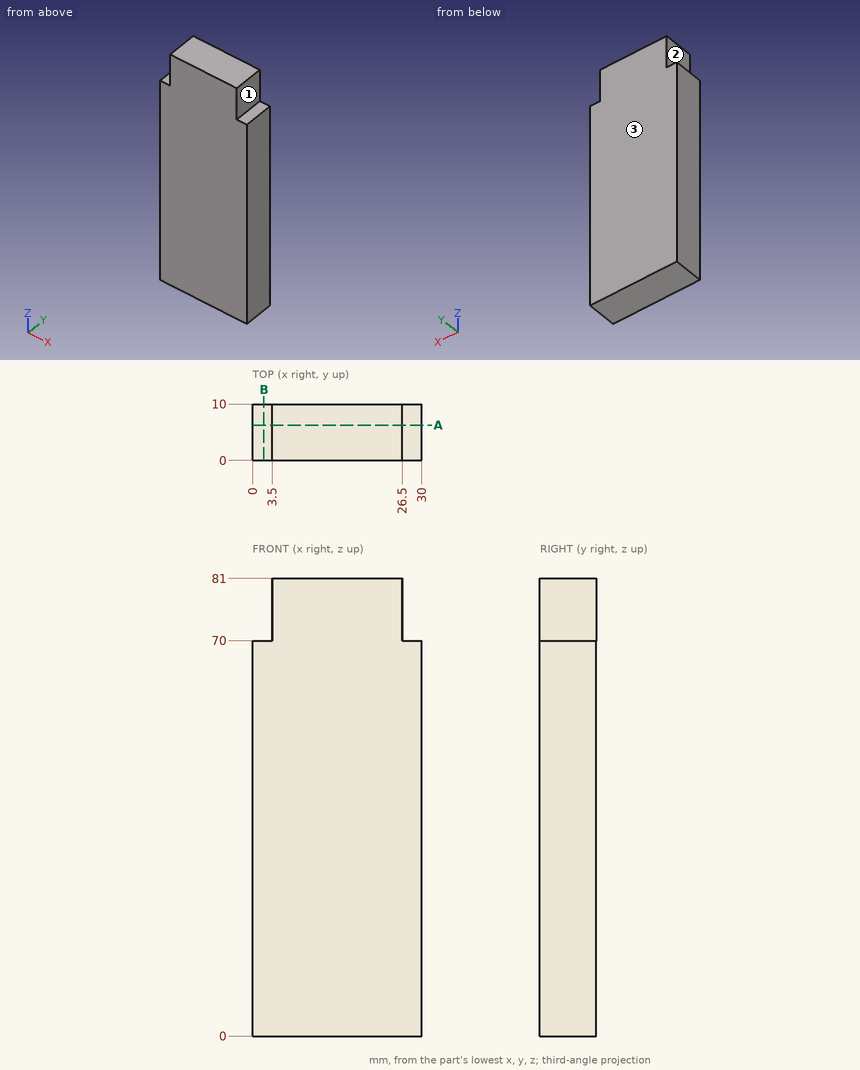
The figure shows three views and two pictorial views of one solid part (mm, origin at its lowest corner). Answer the questions. A direction names the side the tool comes from. Give positions to 0.01 mm unless a question says otherwise; leave off trailing zeros. Loops run counter-clockwise (first coordinate to the right, second up) from the corner with the lowest first, then second, coordinate; pieces in that order, holes last. Notation, with made-up numbers: (-26.5, 74.25) -> (22.5, 74.25) arc R29 ccw to (22.5, 102.25) -> close; hole circle Ø8 at (29.5, 17.5). An arc over 180 degrees is marked (long way). Put each result on its own line as item: value. Start each with the question number.
Item 1: Which of the six approach directions +Z, -Z, +X, -X, +Y, -Y give full straight-line access (tool end or side, diameter ignored) to the marked faces 1, 2 and 3?
Item 2: The part is cut by section A-A (y = 6.25). Give the vertices of the cut face in (x, z), then the cut area to 3 significant figures.
Item 3: Find the intervals of material crossed by L1, parallel to Z at x = 27.5, y = 8.5; L2, parallel to X at y = 3, z = 70.5, in increasing order. Write a range as [from, to].
Item 4: Each of these flat-tipped pins is pushed along its axis until it touches: P1, Ø4, axis at x = 29, y = 3, coming from the +Z side; P2, Ø5, axis at y = 2.5, z = 74, coming from the -X side. Where does it stop, or does it pass through?
Item 5: The part is cut by section B-B (x = 2). Give the vertices of the cut face in (y, z).
Answers below:
1. face 1: +Z, +X, +Y, -Y
1. face 2: +Z, -X, +Y, -Y
1. face 3: +Z, -Z, +X, -X, +Y
2. outline: (0, 0) -> (30, 0) -> (30, 70) -> (26.5, 70) -> (26.5, 81) -> (3.5, 81) -> (3.5, 70) -> (0, 70) -> close
2. area: 2,350 mm2
3. L1: [0, 70]
3. L2: [3.5, 26.5]
4. P1: z = 70
4. P2: x = 3.5
5. outline: (0, 0) -> (10, 0) -> (10, 70) -> (0, 70) -> close
